```python
from build123d import *

# Parameters (mm, degrees)
F0_W     = 1
F0_H     = 1
F1_DEPTH = 3


with BuildPart() as f1:
    # F0 (on Top) → F1 (new body)
    with BuildSketch(Plane.XY):
        Polygon((0, 9.461539), (-10, 9.461539), (-10, 8.461539), (-1, 8.461539), (0, 8.461539), align=None)
        Polygon((10, 9.461539), (0, 9.461539), (0, 8.461539), (1, 8.461539), (10, 8.461539), align=None)
        with Locations((-0.5, 7.961539)):
            Rectangle(F0_W, F0_H)
        with Locations((0.5, 7.961539)):
            Rectangle(F0_W, F0_H)
        Polygon((0, 6.461539), (0, 7.461539), (-1, 7.461539), (-4, 7.461539), (-4, 6.461539), align=None)
        Polygon((1, 7.461539), (0, 7.461539), (0, 6.461539), (4, 6.461539), (4, 7.461539), align=None)
    extrude(amount=F1_DEPTH)


solid = f1.part
```
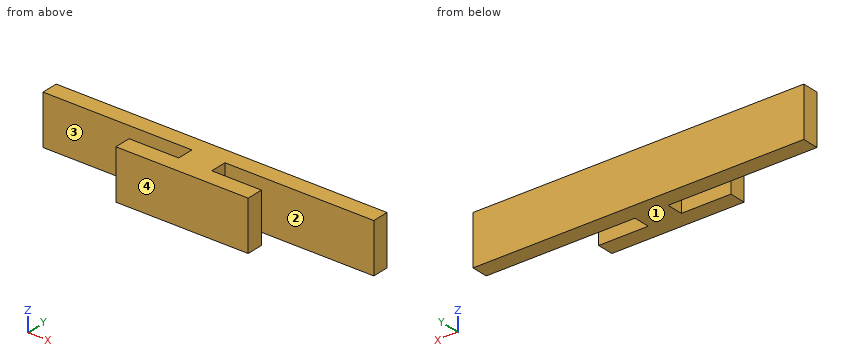
CAD build for the part. Positions are in the model's coordinates, mm. Face numbers are marked on the shaded views. Give positions to 0.01 mm unless a question says otherwise; leave off trailing zeros. Write each loop counter-clockwise with the first axis right and the second up, starting at its lowest first coordinate (ties: lowest second). Pieces come first, ordered by that corner, then holes. Notation, with made-up numbers: M -10,62.5 L 45,62.5 A24 cw 45,81.5 Z; hole C 66,47.25 d11. An arc over 180 degrees is marked long. Return JSON: item names as keys, results as strings. Group by question number.
(1) Band-saw the part on B-B (z = 0.45). Give the cut face in (x, y).
(2) Drill centre lines: L1, parallel to Y at x = 2.5, z = 1.85; L2, parallel to X at y = 8.3, z = 1.25; L3, parallel to Y at x = -6.5, z = 2.7. Where is each one in solid material? Low to high. Write a range as [from, to].
(3) Mould opens along Y. For the marked faces 1, 2, 3 and 4 say: pulls with the +Y half, pulls with the -Y half, needs draft (parallel to the pull), parting line crosses it, or undercut.
(4) Flat gauge pins, fed straight in: pin 1 Ø0.8 at (y, z) = (8, 2) entering from +X; pin 2 Ø0.5 at (y, z) = (7, 1.5) entering from -X. Where does each tip first touch, or does it go through?
(5) Band-saw the part on C-C (y = 7.65). Give the cut face in (x, z).
(6) Band-saw the part on A-A (x = 3). Give the cut face in (y, z), and give its area (3 significant figures).
Entries:
{
 "1": {"outline": "M -10,8.46 L -1,8.46 L -1,7.46 L -4,7.46 L -4,6.46 L 4,6.46 L 4,7.46 L 1,7.46 L 1,8.46 L 10,8.46 L 10,9.46 L -10,9.46 Z"},
 "2": {"L1": "y = [6.46, 7.46], [8.46, 9.46]", "L2": "x = [-1, 1]", "L3": "y = [8.46, 9.46]"},
 "3": {"face 1": "needs draft", "face 2": "undercut", "face 3": "undercut", "face 4": "pulls with the -Y half"},
 "4": {"pin 1": "stops at x = 1", "pin 2": "stops at x = -4"},
 "5": {"outline": "M -1,0 L 1,0 L 1,3 L -1,3 Z"},
 "6": {"outline": "M 6.46,0 L 7.46,0 L 7.46,3 L 6.46,3 Z; M 8.46,0 L 9.46,0 L 9.46,3 L 8.46,3 Z", "area": "6.00 mm^2"}
}
